The listing builds one solid part. Answer for the finished solid, in the listing's coordinates (mm). Face numbers are marked on the shaded views. A direction names the side the tool comes from. Round coordinates to 2 decimals unless told otherwise and drop trailing zeros. Order: outer loops, then holes, each group sorted by start corner. A loop starts at its lowest first (then second) coordinate and runs counter-clockwise, first axis right, second up. Notation, with made-up numbers: M 47,30.25 L 90,30.25 A34 cw 90,69.25 Z; hole C 39.25,-21 d8. An arc over 180 degrees is marked long. Write item = value, one per line. Start each with the question number.
(1) Straight lines are drawn through the part: probe 1 along X at (y, z) = (0.95, 4); probe 2 along Y at (x, z) = (-18.5, 7); probe 3 along Z at (x, y) = (18, 3.1). For each, find the intervals that lie inside material, in ascending order. Write a range as from..to.
(2) Which of the six approach directions +Z, -Z, +X, -X, +Y, -Y give full straight-line access (tool end or side, diameter ignored) to the marked faces 1, 2 and 3?
(3) A cutting plane is placed at D-D, the plane x = -12.5. Determine the outline of the cut face in (y, z), and give its area (3 significant figures).
(4) For a pull along Y with two mould halves and no side action, classify the marked faces 4, 5 and 6 as released by +Y, released by -Y, zero draft, split by the parting line, or undercut.
(5) A cutting plane is placed at C-C, the plane z = 4. Count the separate pieces of the cut face and the enclosed holes in it, and give its area (3 significant figures).
(6) A cutting plane is placed at B-B, the plane y = 2.5. Determine the outline of the cut face in (x, z).
(7) Each of these flat-tipped pins is pushed along its axis until it touches: pin 1 (1.5 mm diameter, centred on y = 22.5, z = 6.5, fed in from +X); pin 2 (2.5 mm diameter, centred on x = 19.5, z = 3.5, fed in from +Y); pin 3 (4 mm diameter, centred on y = 10, z = 1, fed in from +X). Where does it stop, or does it pass through?
(8) A cutting plane is placed at A-A, the plane x = 18. Determine the outline of the cut face in (y, z), and give its area (3 significant figures).
from build123d import *

# Parameters (mm, degrees)
EXTRUDE_1_DEPTH     = 8
SKETCH_2_RX         = 9
SKETCH_2_RY         = 9
CUT_EXTRUDE_1_DEPTH = 37.496575182
FILLET_1_R          = 2
SKETCH_3_R          = 2
CUT_EXTRUDE_2_DEPTH = 37.496575341


with BuildPart() as part:
    # 草图1 → 凸台-拉伸1 (new body)
    with BuildSketch(Plane.XY):
        Polygon((22, 0), (-22, 0), (-22, 4), (-12, 4), (-12, 24), (-22, 24), (-22, 28), (22, 28), (22, 24), (12, 24), (12, 4), (22, 4), align=None)
    extrude(amount=EXTRUDE_1_DEPTH)

    # 草图2 → 切除-拉伸1 (cut, through all)
    with BuildSketch(Plane.XY.offset(8)):
        with Locations(Location((0, 14), (0, 0, 180))):
            Ellipse(SKETCH_2_RX, SKETCH_2_RY)
    extrude(amount=-CUT_EXTRUDE_1_DEPTH, mode=Mode.SUBTRACT)

    # 圆角1
    fillet_1_edges = [part.edges().sort_by_distance(p)[0] for p in [
        (-12, 4, 4),
        (-12, 24, 4),
        (12, 24, 4),
        (12, 4, 4),
    ]]
    fillet(fillet_1_edges, radius=FILLET_1_R)

    # 草图3 → 切除-拉伸2 (cut, through all)
    with BuildSketch(Plane(origin=(0, 28, 0), x_dir=(1, 0, 0), z_dir=(0, 1, 0))):
        with Locations(Location((-18, -4, 0), (0, 0, 270))):
            Circle(SKETCH_3_R)
        with Locations(Location((18, -4, 0), (0, 0, 90))):
            Circle(SKETCH_3_R)
    extrude(amount=-CUT_EXTRUDE_2_DEPTH, mode=Mode.SUBTRACT)


solid = part.part
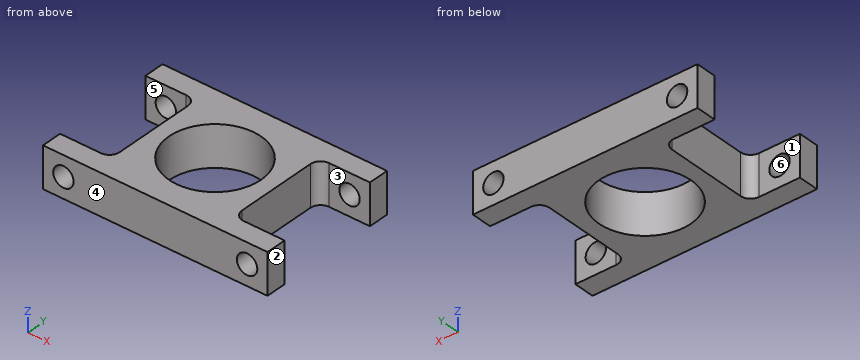
Reported:
q1.probe_1 = -22..-20, -16..16, 20..22
q1.probe_2 = 0..4, 24..28
q1.probe_3 = 0..2, 6..8
q2.face_1 = +Z, -Z, -X
q2.face_2 = +Z, -Z, +X, +Y, -Y
q2.face_3 = +Z, -Z, +X
q3.outline = M 0,0 L 4.68,0 L 4.68,8 L 0,8 Z; M 23.32,0 L 28,0 L 28,8 L 23.32,8 Z
q3.area = 74.8 mm²
q4.face_4 = released by -Y
q4.face_5 = undercut
q4.face_6 = zero draft
q5.separate_pieces = 5
q5.enclosed_holes = 1
q5.area = 517 mm²
q6.outline = M -22,0 L 22,0 L 22,8 L -22,8 Z; hole C -18,4 d4; hole C 18,4 d4
q7.pin_1 = 12.44
q7.pin_2 = 28
q7.pin_3 = 12
q8.outline = M 0,0 L 4,0 L 4,2 L 0,2 Z; M 0,6 L 4,6 L 4,8 L 0,8 Z; M 24,0 L 28,0 L 28,2 L 24,2 Z; M 24,6 L 28,6 L 28,8 L 24,8 Z
q8.area = 32.0 mm²
